Could you check a few things on this drawing? It's one solid part, dimensions in mm from its lowest x, y, z. A direction names the side the tool comes from. Give positions to 0.01 mm unless a question says otherwise; leave off trailing zeros. Loops run counter-clockwise (first coordinate to the right, second up) from the corner with the lowest first, then second, coordinate; pieces in that order, holes last. Notation, with made-up numbers: M -8.5,61 L 36.5,61 A10 cw 36.5,75 Z; hole C 61.25,4 d9. An arc over 180 degrees is marked long. Write each question's results on one line, items separated by ' | '. Start each with the question number.
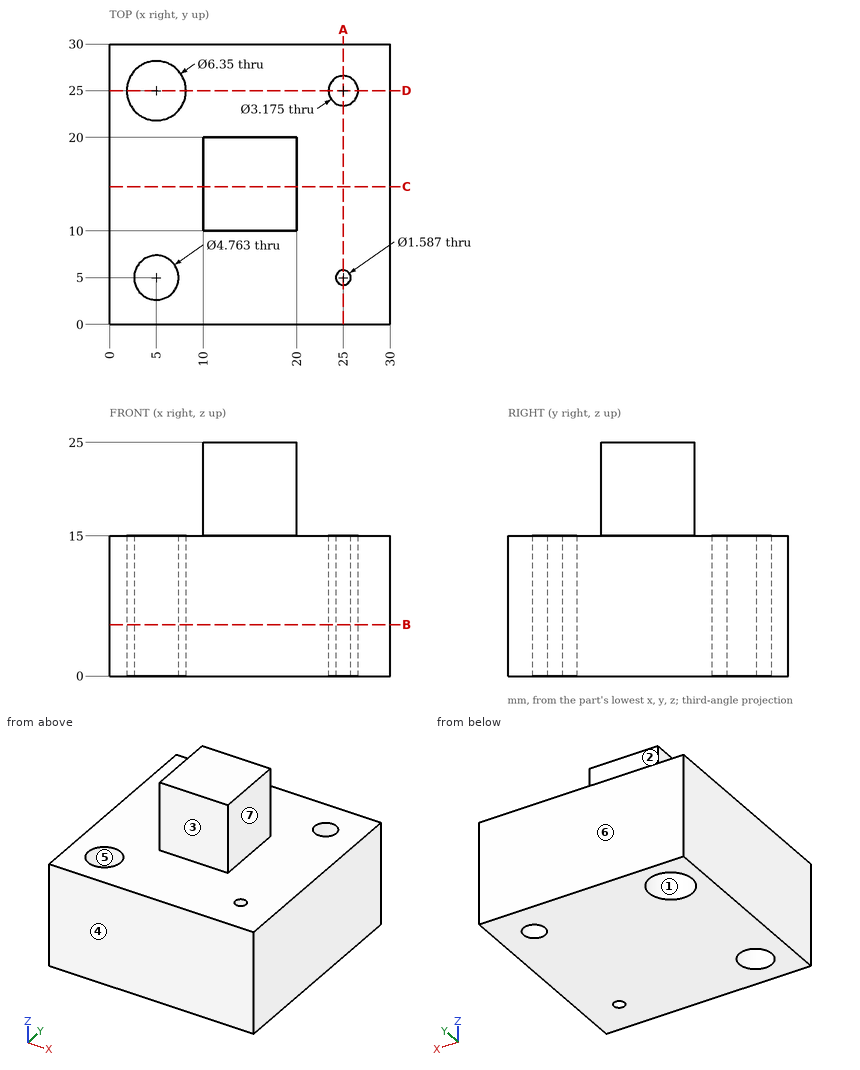
1) Thinking about a two-plate mould opening in Y: for the marked faces 4, 5, 6 and 7, which applies, pulls with the +Y half, pulls with the -Y half, needs draft (parallel to the pull), parting line crosses it, or undercut?
2) If we section it at A-A on x = 25: Write out the boundary of the cut face in (y, z).
3) If we section it at D-D on y = 25: Write out the boundary of the cut face in (x, z) (1 decimal), plus the area to 3 significant figures.
4) I'm going to push flat-ended pins straight in: P1, Ø11, axis at x = 14.5, z = 21, coming from the +Y side; P2, Ø8, axis at y = 16.5, z = 21.5, coming from the +X side; P3, Ø3, axis at x = 15, z = 19.5, coming from the -Y side. Where does each tip first touch, or does it pass through?
5) Please list where these lines run through material, in increasing order: line 1 (Y direction, x = 25, z = 7); line 2 (Y direction, x = 5, z = 8.75) (1 decimal); line 3 (Z direction, x = 7.75, y = 17.5). Write a range as from..to.
6) If we section it at C-C on y = 14.75: Write out the boundary of the cut face in (x, z), plus the area to 3 significant figures.
7) If we section it at B-B on z = 5.5: State how many separate pieces and enclosed holes the cut face has.
8) Which directions (+Z, -Z, +X, -X, +Y, -Y) give clear straight access to the entire face, cutting with the end or side of a thin tool? Please do the marked faces 1, 2 and 3.
Calculated:
1) face 4: pulls with the -Y half | face 5: undercut | face 6: pulls with the +Y half | face 7: needs draft
2) outline: M 0,0 L 4.21,0 L 4.21,15 L 0,15 Z; M 5.79,0 L 23.41,0 L 23.41,15 L 5.79,15 Z; M 26.59,0 L 30,0 L 30,15 L 26.59,15 Z
3) outline: M 0,0 L 1.8,0 L 1.8,15 L 0,15 Z; M 8.2,0 L 23.4,0 L 23.4,15 L 8.2,15 Z; M 26.6,0 L 30,0 L 30,15 L 26.6,15 Z | area: 307 mm2
4) P1: stops at y = 20 | P2: stops at x = 20 | P3: stops at y = 10
5) line 1: y = 0..4.21, 5.79..23.41, 26.59..30 | line 2: y = 0..2.6, 7.4..21.8, 28.2..30 | line 3: z = 0..15
6) outline: M 0,0 L 30,0 L 30,15 L 20,15 L 20,25 L 10,25 L 10,15 L 0,15 Z | area: 550 mm2
7) separate pieces: 1 | enclosed holes: 4
8) face 1: +Z, -Z | face 2: +Z, +X, -X, +Y | face 3: +Z, +X, -X, -Y
